Design review of the part built by this model. Coordinates are the model's own, in mm. A direction names the side the tool comes from. Coordinates: 2 decimals unless noted, no trailing zeros. Write each loop counter-clockwise with the first axis right and the second up, starting at its lowest first coordinate (ties: lowest second). Pieces come first, ordered by that corner, then holes. Notation, with made-up numbers: (40.5, 20) -> (53.5, 20) arc R37 cw to (53.5, 56) -> close; hole circle Ø11 at (34.25, 48.25). An arc over 180 degrees is marked (long way). Answer in a Markdown table with one row per item. Add a question column.
Item 1: Take a section at C-C, the plane x = 92.5. Write out the cut boundary in (y, z), and give its area (3 significant figures).
Item 2: To check wall thickness, follow line 1 (X direction, y = -6, z = 17); line 2 (Y direction, x = 55, z = 11.75); line 3 (Z direction, x = 192.5, y = 50.5). State the ranges of each line that lie inside material, in increasing order.
Item 3: Draft analysis for pull direction X (two halves, no side actions). For faces 1 (the face through (200, -1, 16)), 2 (the face through (41, -1, 1.964)), 3 (the face through (99, 77.5, 16)), 4 (the face through (99, -1, 0)), state which applies: released by +X, released by -X, zero draft, split by the parting line, or undercut.
Item 4: Take a section at A-A, the plane z = 21.5. Write out the cut boundary in (x, y).
Item 5: Clearance check with flat-ended pins moving along their axes: P1, Ø10, axis at x = 105, y = 61.5, coming from the +Z side; P2, Ø1.3, axis at x = 82.5, y = 38.5, coming from the +Z side. State where each tip first meets the part, or that it passes through.
Item 6: Take a section at B-B, the plane y = 10.5. Write out the cut boundary in (x, z), and give its area (3 significant figures).
Item 7: For faces 5 (the face through (99, 80, 17)), 6 (the face through (1.665, -1, 16)), list the 3-axis set-ups (+Z, -Z, +X, -X, +Y, -Y) from which the entire face can be reached by the end or side of a thin tool; tool diameter is ignored.
from build123d import *

# Parameters (mm, degrees)
F0_W     = 200
F0_H     = 30
F1_DEPTH = 80
F2_W     = 0.6549034361
F2_H     = 3.5952763587
F2_W_2   = 1.654828703
F2_W_3   = 2.3097321391
F3_DEPTH = 77.5
F4_SIZE  = 3


with BuildPart() as f1:
    # F0 (on Front) → F1 (new body, symmetric)
    with BuildSketch(Plane.XZ):
        with Locations((100, 15)):
            Rectangle(F0_W, F0_H)
    extrude(amount=F1_DEPTH, both=True)

    # F2 (on Front) → F3 (cut, symmetric)
    with BuildSketch(Plane.XZ):
        Polygon((81.0098946095, 30.9638166718), (1.6647980455, 30.9638166718), (1.6647980455, 1.9638166718), (81.6647980455, 1.9638166718), (81.6647980455, 27.3685403131), (81.0098946095, 27.3685403131), align=None)
        with Locations((81.3373463275, 29.1661784924)):
            Rectangle(F2_W, F2_H)
        with Locations((82.492212397, 29.1661784924)):
            Rectangle(F2_W_2, F2_H)
        with Locations((84.4744928181, 29.1661784924)):
            Rectangle(F2_W_3, F2_H)
        Polygon((85.6293588877, 27.3685403131), (83.3196267486, 27.3685403131), (83.3196267486, 1.9638166718), (198.3196267486, 1.9638166718), (198.3196267486, 30.9638166718), (85.6293588877, 30.9638166718), align=None)
    extrude(amount=F3_DEPTH, both=True, mode=Mode.SUBTRACT)

    # F4
    f4_edges = [f1.edges().sort_by_distance(p)[0] for p in [
        (100, -80, 0),
        (0, 0, 0),
        (100, 80, 0),
        (200, 0, 0),
    ]]
    chamfer(f4_edges, length=F4_SIZE)


solid = f1.part
Answers:
| question | item | result |
|---|---|---|
| 1 | outline | (-80, 3) -> (-77, 0) -> (77, 0) -> (80, 3) -> (80, 30) -> (77.5, 30) -> (77.5, 1.96) -> (-77.5, 1.96) -> (-77.5, 30) -> (-80, 30) -> close |
| 1 | area | 445 mm^2 |
| 2 | line 1 | x = 0 to 1.66, 81.66 to 83.32, 198.32 to 200 |
| 2 | line 2 | y = -80 to -77.5, 77.5 to 80 |
| 2 | line 3 | z = 0 to 1.96 |
| 3 | face 1 | released by +X |
| 3 | face 2 | undercut |
| 3 | face 3 | undercut |
| 3 | face 4 | zero draft |
| 4 | outline | (0, -80) -> (200, -80) -> (200, 80) -> (0, 80) -> close; hole (1.66, -77.5) -> (81.66, -77.5) -> (81.66, 77.5) -> (1.66, 77.5) -> close; hole (83.32, -77.5) -> (198.32, -77.5) -> (198.32, 77.5) -> (83.32, 77.5) -> close |
| 5 | P1 | stops at z = 1.96 |
| 5 | P2 | stops at z = 27.37 |
| 6 | outline | (0, 3) -> (3, 0) -> (197, 0) -> (200, 3) -> (200, 30) -> (198.32, 30) -> (198.32, 1.96) -> (83.32, 1.96) -> (83.32, 27.37) -> (81.66, 27.37) -> (81.66, 1.96) -> (1.66, 1.96) -> (1.66, 30) -> (0, 30) -> close |
| 6 | area | 520 mm^2 |
| 7 | face 5 | +Z, -Z, +X, -X, +Y |
| 7 | face 6 | +Z |
